Input: dimensioned drawing with shaded views. Units: mm. Origin: part minimum x, y, z. A direction names the side the tool comes from. Round coordinates to 2 decimals unless told otherwise and drop trailing zeros. Order: outer loops, then holes, each group sorted by start corner. A loop starts at its lowest first (then second) coordinate and runs counter-clockwise, first axis right, second up. Notation, with made-up numbers: (-8.75, 9.25) - (45.25, 9.25) arc R17 ccw to (45.25, 13.25) - close; hole circle Ø1 at (49.5, 16.25). An arc over 180 degrees is marked (long way). Return JSON: item names as keys, results as strings. Group by question number.
1) Section D-D, the plane y = 52.5. Return loops of the section in (x, z).
2) Contact query for flat-ended pins moving along their axis: P1, Ø5, axis at y = 58, z = 6, coming from the -X side; P2, Ø5, axis at y = 61, z = 6, coming from the +X side; P3, Ø3, axis at x = 56.5, z = 6.5, coming from the +Y side. Output: stop coordinate, or through.
3) Access query for the marked faces 4, 5 and 6. Directions: +Z, -Z, +X, -X, +Y, -Y. A direction counts if a zero-diameter tool reaches every point of the face in a straight line with its end or side. Return the directions, or none.
4) Ray query, line 1 (Y direction, x = 30, z = 7); line 2 (Y direction, x = 28, z = 7.25); line 3 (X direction, y = 77, z = 5.25) (3 decimals). Return the intervals inside material, ascending. Write a range as from..to.
5) Section C-C, the plane y = 73.5. Return loops of the section in (x, z).
6) Section B-B, the plane z = 3.25. Return loops of the section in (x, y), plus the area to 3 significant figures.
7) Section A-A, the plane x = 30. Return loops of the section in (y, z).
8) Mould query, pull axis Y, two halves, no side actions, for the marked faces 1, 2 and 3. Classes: pulls with the +Y half, pulls with the -Y half, needs draft (parallel to the pull), parting line crosses it, or undercut.
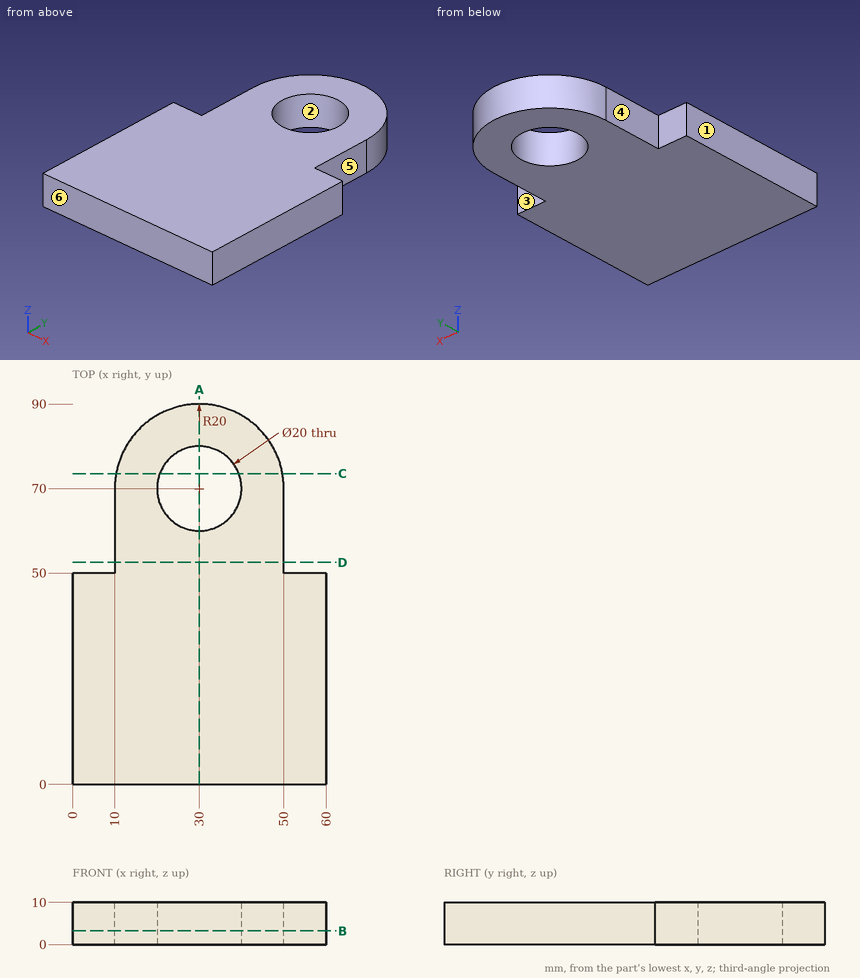
Geometry check:
{
 "1": {"outline": "(10, 0) - (50, 0) - (50, 10) - (10, 10) - close"},
 "2": {"P1": "x = 10", "P2": "x = 50", "P3": "y = 50"},
 "3": {"face 4": "+Z, -Z, -X, +Y", "face 5": "+Z, -Z, +X, +Y", "face 6": "+Z, -Z, +X, -X, -Y"},
 "4": {"line 1": "0..60, 80..90", "line 2": "0..60.2, 79.8..89.9", "line 3": "11.265..22.859, 37.141..48.735"},
 "5": {"outline": "(10.31, 0) - (20.63, 0) - (20.63, 10) - (10.31, 10) - close; (39.37, 0) - (49.69, 0) - (49.69, 10) - (39.37, 10) - close"},
 "6": {"outline": "(0, 0) - (60, 0) - (60, 50) - (50, 50) - (50, 70) arc R20 ccw to (10, 70) - (10, 50) - (0, 50) - close; hole circle Ø20 at (30, 70)", "area": "4,110 mm2"},
 "7": {"outline": "(0, 0) - (60, 0) - (60, 10) - (0, 10) - close; (80, 0) - (90, 0) - (90, 10) - (80, 10) - close"},
 "8": {"face 1": "needs draft", "face 2": "undercut", "face 3": "pulls with the +Y half"}
}
